Autodesk Inventor part; units mm, degrees
ref_plane "YZ Plane" through (0, 0, 0) normal (1, 0, 0) x (0, 1, 0)
ref_plane "XZ Plane" through (0, 0, 0) normal (0, 1, 0) x (-1, 0, 0)
ref_plane "XY Plane" through (0, 0, 0) normal (0, 0, 1) x (1, 0, 0)
sketch "Sketch1" plane through (0, 0, 0) normal (0, 0, 1) x (1, 0, 0)
  line L0 (-43.0288, 68.3746) -> (111.0984, 68.3746)
  line L1 (111.0984, 68.3746) -> (111.0984, -111.7622)
  line L2 (111.0984, -111.7622) -> (-43.0288, -111.7622)
  line L3 (-43.0288, -111.7622) -> (-43.0288, 68.3746)
  line L4 (111.0984, 68.3746) -> (111.0984, 28.3696)
  line L5 (-43.0288, 68.3746) -> (-36.0288, 68.3746)
  line L6 (111.0984, 68.3746) -> (104.0984, 68.3746)
  line L7 (111.0984, -111.7622) -> (111.0984, -71.7572)
  line L8 (111.0984, 68.3746) -> (111.0984, 38.3746)
  line L9 (111.0984, -111.7622) -> (111.0984, -81.7622)
  circle A0 centre (104.0984, 38.3746) radius 3.5
  circle A1 centre (104.0984, -81.7622) radius 3.5
  circle A2 centre (-36.0288, 38.3746) radius 3.5
  circle A3 centre (-36.0288, -81.7622) radius 3.5
  circle A4 centre (-15.9652, -6.6938) radius 2.0193
  circle A5 centre (-15.9652, -36.6938) radius 2.0193
  circle A6 centre (84.0348, -36.6938) radius 2.0193
  circle A7 centre (84.0348, -6.6938) radius 2.0193
  point P0 (0, 0)
  dimension "d0" = 154.1272
  dimension "d1" = 180.1368
  dimension "d3" = 7
  dimension "d4" = 7
  dimension "d30" = 30
  dimension "d31" = 30
  dimension "d32" = 7
  dimension "d33" = 7
  dimension "d38" = 4.0386
  dimension "d39" = 4.0386
  dimension "d40" = 4.0386
  dimension "d41" = 4.0386
extrude "Extrusion1" add sketch "Sketch1" along normal blind 6.35
properties part number "xy axis mount"
Geometry check sheet. Reference: the model listing, model coordinates, mm. Coordinates: 2 decimals unless noted, no trailing zeros. Answer as a JSON object with one key per item and string values. Group by question number.
Item 1: Draft check along X on faces 1 (the face through (33, -20, 0)), 2 (the face through (-14.88, -8.396, 3.131)), 3 (the face through (-43.029, -23, 3)). Enter one of: +X half, -X half, draft (parallel to the pull), parting line (faces both ways), or undercut.
Item 2: Scan lines: probe 1 along Y at (x, z) = (83, 5.75); probe 2 along X at (y, z) = (35.5, 0.5). Record each from-to range of solid material in increasing order.
Item 3: Depth check by flat-ended pin: pin 1 Ø4 at (x, y) = (104.1, 38.37) entering from -Z. Enter the tip coordinate at first touch or a pass-through.
Resolved:
{
 "1": {"face 1": "draft", "face 2": "undercut", "face 3": "-X half"},
 "2": {"probe 1": "-111.76 to -38.43, -34.96 to -8.43, -4.96 to 68.37", "probe 2": "-43.03 to -38.03, -34.03 to 102.1, 106.1 to 111.1"},
 "3": {"pin 1": "through"}
}
